from build123d import *

# Parameters (mm, degrees)
SKETCH1_R            = 8.509
BOSS_EXTRUDE1_DEPTH  = 3.81
SKETCH3_W            = 7.9375
SKETCH3_H            = 5.08
CUT_EXTRUDE2_DEPTH   = 3.81
M2_CLEARANCE_HOLE1_D = 2.4
FILLET1_R            = 1.5875


with BuildPart() as part:
    # Sketch1 → Boss-Extrude1 (new body)
    with BuildSketch(Plane.XY):
        Circle(SKETCH1_R)
    extrude(amount=BOSS_EXTRUDE1_DEPTH)

    # Sketch3 → Cut-Extrude2 (cut)
    with BuildSketch(Plane.XY.offset(3.81)):
        Rectangle(SKETCH3_W, SKETCH3_H)
    extrude(amount=-CUT_EXTRUDE2_DEPTH, mode=Mode.SUBTRACT)

    # M2 Clearance Hole1 (through all)
    with Locations(Plane.XY.offset(3.81)):
        with Locations((-6.223, 0), (3.1115, 5.389276088), (3.1115, -5.389276088)):
            Hole(M2_CLEARANCE_HOLE1_D / 2)

    # Fillet1
    fillet1_edges = [part.edges().sort_by_distance(p)[0] for p in [
        (3.96875, 2.54, 1.905),
        (3.96875, -2.54, 1.905),
        (-3.96875, -2.54, 1.905),
        (-3.96875, 2.54, 1.905),
    ]]
    fillet(fillet1_edges, radius=FILLET1_R)


solid = part.part
Can you work these out from the model? Positions are in its coordinate system, mm. A direction names the side the tool comes from. Give positions to 0.01 mm unless a question says otherwise; leave off trailing zeros. Order: outer loops, then holes, each group sorted by start corner. A loop starts at its lowest first (then second) coordinate and runs counter-clockwise, first axis right, second up. Notation, with made-up numbers: M 54,88 L 100,88 A12 cw 100,94 Z; hole C -29,53 d5. An arc over 180 degrees is marked long. Use one line per item in the form item = value.
Item 1: If we section it at C-C, the plane y = 2: Write out the boundary of the cut face in (x, z), and give its area (3 significant figures).
Values follow:
outline = M -8.27,0 L -3.57,0 L -3.57,3.81 L -8.27,3.81 Z; M 3.57,0 L 8.27,0 L 8.27,3.81 L 3.57,3.81 Z
area = 35.8 mm^2
Item 2: If we section it at B-B, the plane x = 0: Write out the boundary of the cut face in (y, z).
Values follow:
outline = M -8.51,0 L -2.54,0 L -2.54,3.81 L -8.51,3.81 Z; M 2.54,0 L 8.51,0 L 8.51,3.81 L 2.54,3.81 Z
Item 3: If we section it at D-D, the plane z = 0.4: Write out the boundary of the cut face in (x, y) (1 decimal), and give its area (3 significant figures).
Values follow:
outline = C 0,0 d17; hole C -6.2,0 d2.4; hole M -4,-1 A1.6 ccw -2.4,-2.5 L 2.4,-2.5 A1.6 ccw 4,-1 L 4,1 A1.6 ccw 2.4,2.5 L -2.4,2.5 A1.6 ccw -4,1 Z; hole C 3.1,-5.4 d2.4; hole C 3.1,5.4 d2.4
area = 176 mm^2
Item 4: If I drill on line 1 along X through (y, z) = (0.5, 1.75); line 2 along Y through (x, z) = (4, 1.45); line 3 along X through (y, z) = (-2.25, 2.9), over which ranges is the centre line in solid material (lowest first)? Write a range as [from, to].
Values follow:
line_1 = [-8.49, -7.31], [-5.13, -3.97], [3.97, 8.49]
line_2 = [-7.51, -6.2], [-4.58, 4.58], [6.2, 7.51]
line_3 = [-8.21, -3.3], [3.3, 8.21]
Item 5: If we section it at A-A, the plane y = 0: Write out the boundary of the cut face in (x, z), and give its area (3 significant figures).
Values follow:
outline = M -8.51,0 L -7.42,0 L -7.42,3.81 L -8.51,3.81 Z; M -5.02,0 L -3.97,0 L -3.97,3.81 L -5.02,3.81 Z; M 3.97,0 L 8.51,0 L 8.51,3.81 L 3.97,3.81 Z
area = 25.5 mm^2
Item 6: Thinking about a two-plate mould opening in Y: for faces 3 (the cylindrical face through (2.558, 4.325, 1.878)), 4 (the cylindrical face through (-1.108, 8.437, 1.878)), 5 (the flat face through (0, -4, 3.81)), which applies, pulls with the +Y half, pulls with the -Y half, needs draft (parallel to the pull), parting line crosses it, or undercut?
Values follow:
face_3 = undercut
face_4 = parting line crosses it
face_5 = needs draft
Item 7: For faces 1 (the cylindrical face through (-3.49, -2.09, 1.88)), 2 (the flat face through (0, -4, 0)), which set-ups out of +Z, -Z, +X, -X, +Y, -Y let a thin tool reach every point of the face, with its end or its side?
Values follow:
face_1 = +Z, -Z
face_2 = -Z, +X, -X, +Y, -Y
Item 8: Will these pins go through, and if not, where does the flat tip stop? pin 1 Ø3 at (x, y) = (3.11, -5.39) entering from -Z; pin 2 Ø1.9 at (x, y) = (-6.223, 0) entering from +Z; pin 3 Ø1 at (x, z) = (3.5, 3.5) entering from +Y.
Values follow:
pin_1 = 0
pin_2 = through
pin_3 = 7.96
